Build history of the part. All positions in model axes, mm. A direction names the side the tool comes from. Coordinates: 2 decimals unless noted, no trailing zeros. Order: outer loops, then holes, each group sorted by start corner. A loop starts at its lowest first (then second) coordinate and runs counter-clockwise, first axis right, second up. Notation, with made-up numbers: M -28,51.25 L -11,51.25 A7 ccw -11,56.25 Z; hole C 3,49 d8. An arc over 180 degrees is marked long. Use a Markdown table: item, result. Add a question column.
from build123d import *

# Parameters (mm, degrees)
F0_W     = 50
F0_H     = 3
F0_W_2   = 21.25
F1_DEPTH = 3
F2_DEPTH = 2


with BuildPart() as f1:
    # F0 (on Front) → F1 (new body)
    with BuildSketch(Plane.XZ):
        with BuildLine():
            ThreePointArc((50.233181265, -1.3), (50.2457951403, -0.6500543958), (50.25, 0))
            ThreePointArc((50.25, 0), (50.2457951403, 0.6500543958), (50.233181265, 1.3))
            Line((50.233181265, 1.3), (46.25, 1.3))
            Line((46.25, 1.3), (46.25, -1.3))
            Line((46.25, -1.3), (50.233181265, -1.3))
        make_face()
        with BuildLine():
            Line((46.25, 1.3), (50.233181265, 1.3))
            ThreePointArc((50.233181265, 1.3), (50.171859503, 2.8012522223), (50.0656818589, 4.3))
            Line((50.0656818589, 4.3), (46.25, 4.3))
            Line((46.25, 4.3), (46.25, 1.3))
        make_face()
        with BuildLine():
            ThreePointArc((50.0656818589, -4.3), (50.171859503, -2.8012522223), (50.233181265, -1.3))
            Line((50.233181265, -1.3), (46.25, -1.3))
            Line((46.25, -1.3), (46.25, -4.3))
            Line((46.25, -4.3), (50.0656818589, -4.3))
        make_face()
        with BuildLine():
            Line((46.25, 4.3), (50.0656818589, 4.3))
            ThreePointArc((50.0656818589, 4.3), (0, 50.25), (-50.0656818589, 4.3))
            Line((-50.0656818589, 4.3), (-46.25, 4.3))
            Line((-46.25, 4.3), (-25, 4.3))
            Line((-25, 4.3), (25, 4.3))
            Line((25, 4.3), (46.25, 4.3))
        make_face()
        with BuildLine():
            ThreePointArc((-50.0656818589, -4.3), (0, -50.25), (50.0656818589, -4.3))
            Line((50.0656818589, -4.3), (46.25, -4.3))
            Line((46.25, -4.3), (25, -4.3))
            Line((25, -4.3), (-25, -4.3))
            Line((-25, -4.3), (-46.25, -4.3))
            Line((-46.25, -4.3), (-50.0656818589, -4.3))
        make_face()
        with BuildLine():
            Line((-46.25, 4.3), (-50.0656818589, 4.3))
            ThreePointArc((-50.0656818589, 4.3), (-50.171859503, 2.8012522223), (-50.233181265, 1.3))
            Line((-50.233181265, 1.3), (-46.25, 1.3))
            Line((-46.25, 1.3), (-46.25, 4.3))
        make_face()
        with BuildLine():
            ThreePointArc((-50.233181265, -1.3), (-50.171859503, -2.8012522223), (-50.0656818589, -4.3))
            Line((-50.0656818589, -4.3), (-46.25, -4.3))
            Line((-46.25, -4.3), (-46.25, -1.3))
            Line((-46.25, -1.3), (-50.233181265, -1.3))
        make_face()
        with BuildLine():
            Line((-46.25, 1.3), (-50.233181265, 1.3))
            ThreePointArc((-50.233181265, 1.3), (-50.25, 0), (-50.233181265, -1.3))
            Line((-50.233181265, -1.3), (-46.25, -1.3))
            Line((-46.25, -1.3), (-46.25, 1.3))
        make_face()
        with Locations((0, -2.8)):
            Rectangle(F0_W, F0_H)
        with Locations((0, 2.8)):
            Rectangle(F0_W, F0_H)
        with Locations((-35.625, 2.8)):
            Rectangle(F0_W_2, F0_H)
        with Locations((35.625, 2.8)):
            Rectangle(F0_W_2, F0_H)
        with Locations((35.625, -2.8)):
            Rectangle(F0_W_2, F0_H)
        with Locations((-35.625, -2.8)):
            Rectangle(F0_W_2, F0_H)
    extrude(amount=F1_DEPTH)

    # F0 (on Front) → F2 (join)
    with BuildSketch(Plane.XZ):
        with Locations((0, -2.8)):
            Rectangle(F0_W, F0_H)
        with Locations((0, 2.8)):
            Rectangle(F0_W, F0_H)
        with Locations((35.625, -2.8)):
            Rectangle(F0_W_2, F0_H)
        with Locations((35.625, 2.8)):
            Rectangle(F0_W_2, F0_H)
        with Locations((-35.625, 2.8)):
            Rectangle(F0_W_2, F0_H)
        with Locations((-35.625, -2.8)):
            Rectangle(F0_W_2, F0_H)
    extrude(amount=-F2_DEPTH)


solid = f1.part
(1) Slice it at C-C on x = 33.5. Give the cut face in (y, z).
(2) Which spindle directions (+Z, -Z, +X, -X, +Y, -Y) get a long thin tool onto all of the face, cutting with end or side? Do faces 4 (the flat face through (46.25, -1, 0)), 5 (the flat face through (-1, -3, -10)). Say none if no direction does.
(3) Drill centre lines: line 1 along Z through (x, y) = (4, -2.7); line 2 along Z through (x, y) = (1, 1.25); line 3 along Y through (x, z) = (-7.5, -22). Where is each one in solid material? Low to high. Write a range as from..to.
(4) Slice it at B-B on x = 4. Give the cut face in (y, z), and give its area (3 significant figures).
(5) Drop flat-ended pins along their axis: P1, Ø1.6, axis at y = 1.5, z = -2.5, coming from the +X side; P2, Ø1.5, axis at x = 12.5, y = -1.5, coming from the -Z side; P3, Ø1.5, axis at y = 0.5, z = -36, coming from the -X side. Give the stop position or say it passes through.
(6) Mould opens along Z. For faces 1 (the flat face through (-1, 2, 3)), 2 (the flat face through (1, -1, -1.3)), 3 (the flat face through (-46.25, -1, 0)) say: released by +Z, released by -Z, zero draft, split by the parting line, or undercut.
(7) Slice it at A-A on y = -1.1. Give the cut face in (x, z), and give its area (3 significant figures).
(8) Slice it at D-D on z = -22. Give the cut face in (x, y).
Solutions:
| question | item | result |
|---|---|---|
| 1 | outline | M -3,-37.45 L 0,-37.45 L 0,-4.3 L 2,-4.3 L 2,-1.3 L -3,-1.3 Z; M -3,1.3 L 2,1.3 L 2,4.3 L 0,4.3 L 0,37.45 L -3,37.45 Z |
| 2 | face 4 | +Y, -Y |
| 2 | face 5 | +Z, -Z, +X, -X, -Y |
| 3 | line 1 | -50.09..-1.3, 1.3..50.09 |
| 3 | line 2 | -4.3..-1.3, 1.3..4.3 |
| 3 | line 3 | -3..0 |
| 4 | outline | M -3,-50.09 L 0,-50.09 L 0,-4.3 L 2,-4.3 L 2,-1.3 L -3,-1.3 Z; M -3,1.3 L 2,1.3 L 2,4.3 L 0,4.3 L 0,50.09 L -3,50.09 Z |
| 4 | area | 305 mm² |
| 5 | P1 | x = 46.25 |
| 5 | P2 | z = -48.86 |
| 5 | P3 | x = -35.62 |
| 6 | face 1 | zero draft |
| 6 | face 2 | undercut |
| 6 | face 3 | undercut |
| 7 | outline | C 0,0 d100.5; hole M -46.25,-1.3 L 46.25,-1.3 L 46.25,1.3 L -46.25,1.3 Z |
| 7 | area | 7,690 mm² |
| 8 | outline | M -45.18,-3 L 45.18,-3 L 45.18,0 L -45.18,0 Z |
